Read the model definition and answer for the solid it produces. Units are mm, in the model's axes. Give positions to 0.01 mm unless a question says otherwise; leave off trailing zeros. Order: outer loops, then holes, each group sorted by start corner. A loop starts at its lowest first (then second) coordinate and runs counter-clockwise, first axis right, second up. Notation, with made-up numbers: M 66.5,13.25 L 90.5,13.25 A12 cw 90.5,24.25 Z; hole C 0,27 d6. An arc over 180 degrees is marked long. One line per item, written item: value.
from build123d import *

# Parameters (mm, degrees)
SKETCH1_W           = 210
SKETCH1_H           = 30
BOSS_EXTRUDE1_DEPTH = 3
SKETCH2_W           = 50
SKETCH2_H           = 3
BOSS_EXTRUDE2_DEPTH = 3
SKETCH3_R           = 8.15
CUT_EXTRUDE1_DEPTH  = 10
SKETCH4_R           = 2.5
CUT_EXTRUDE2_DEPTH  = 10


with BuildPart() as part:
    # Sketch1 → Boss-Extrude1 (new body)
    with BuildSketch(Plane(origin=(0, 0, 0), x_dir=(1, 0, 0), z_dir=(0, 1, 0))):
        Rectangle(SKETCH1_W, SKETCH1_H)
    extrude(amount=BOSS_EXTRUDE1_DEPTH)

    # Sketch2 → Boss-Extrude2 (add)
    with BuildSketch(Plane(origin=(0, 0, 0), x_dir=(1, 0, 0), z_dir=(0, 1, 0))):
        with Locations((-50, 16.5)):
            Rectangle(SKETCH2_W, SKETCH2_H)
        with Locations((50, 16.5)):
            Rectangle(SKETCH2_W, SKETCH2_H)
        with Locations((50, -16.5)):
            Rectangle(SKETCH2_W, SKETCH2_H)
        with Locations((-50, -16.5)):
            Rectangle(SKETCH2_W, SKETCH2_H)
    extrude(amount=BOSS_EXTRUDE2_DEPTH)

    # Sketch3 → Cut-Extrude1 (cut)
    with BuildSketch(Plane(origin=(0, 3, 0), x_dir=(1, 0, 0), z_dir=(0, 1, 0))):
        with Locations(Location((-12.7, 0, 0), (0, 0, 270))):
            Circle(SKETCH3_R)
        with Locations(Location((12.7, 0, 0), (0, 0, 90))):
            Circle(SKETCH3_R)
    extrude(amount=-CUT_EXTRUDE1_DEPTH, mode=Mode.SUBTRACT)

    # Sketch4 → Cut-Extrude2 (cut)
    with BuildSketch(Plane(origin=(0, 3, 0), x_dir=(1, 0, 0), z_dir=(0, 1, 0))):
        with Locations(Location((-95, 0, 0), (0, 0, 270))):
            Circle(SKETCH4_R)
        with Locations(Location((-87.5, 5, 0), (0, 0, 270))):
            Circle(SKETCH4_R)
        with Locations(Location((-87.5, -5, 0), (0, 0, 270))):
            Circle(SKETCH4_R)
        with Locations(Location((87.5, -5, 0), (0, 0, 90))):
            Circle(SKETCH4_R)
        with Locations(Location((87.5, 5, 0), (0, 0, 90))):
            Circle(SKETCH4_R)
        with Locations(Location((95, 0, 0), (0, 0, 90))):
            Circle(SKETCH4_R)
    extrude(amount=-CUT_EXTRUDE2_DEPTH, mode=Mode.SUBTRACT)


solid = part.part
1) Consider probe 1 along X at (y, z) = (1.9, 0); probe 2 along Z at (x, y) = (87.5, 1.3); probe 3 along X at (y, z) = (1.6, 16.5). Determine where each line is inside the solid, lowest interval first.
Reported:
probe 1: x = -105 to -97.5, -92.5 to -20.85, -4.55 to 4.55, 20.85 to 92.5, 97.5 to 105
probe 2: z = -15 to -7.5, -2.5 to 2.5, 7.5 to 15
probe 3: x = -75 to -25, 25 to 75
2) Find section B-B, the plane x = 87.5. Write down the section's boundary in (y, z).
Reported:
outline: M 0,-15 L 3,-15 L 3,-7.5 L 0,-7.5 Z; M 0,-2.5 L 3,-2.5 L 3,2.5 L 0,2.5 Z; M 0,7.5 L 3,7.5 L 3,15 L 0,15 Z
3) Find section A-A, the plane x = 12.7. Write down the section's boundary in (y, z), plus the area to 3 significant figures.
Reported:
outline: M 0,-15 L 3,-15 L 3,-8.15 L 0,-8.15 Z; M 0,8.15 L 3,8.15 L 3,15 L 0,15 Z
area: 41.1 mm^2
4) Find section D-D, the plane z = 5. Write down the section's boundary in (x, y).
Reported:
outline: M -105,0 L -90,0 L -90,3 L -105,3 Z; M -85,0 L -19.14,0 L -19.14,3 L -85,3 Z; M -6.26,0 L 6.26,0 L 6.26,3 L -6.26,3 Z; M 19.14,0 L 85,0 L 85,3 L 19.14,3 Z; M 90,0 L 105,0 L 105,3 L 90,3 Z
5) Find section C-C, the plane y = 2.15. Count the separate pieces of the cut face and the enclosed holes in it, plus the area to 3 significant figures.
Reported:
separate pieces: 1
enclosed holes: 8
area: 6,360 mm^2
6) Determine the mould class of faces 1 (the face through (-1, 3, 0)), 2 (the face through (-5.828, 1.521, 4.381)) for opening direction X: +X half, -X half, draft (parallel to the pull), parting line (faces both ways), or undercut.
Reported:
face 1: draft
face 2: undercut
7) Each of these flat-tipped pins is pushed along its axis until it touches: pin 1 Ø1.5 at (x, y) = (92.5, 2) entering from -Z; pin 2 Ø4 at (x, z) = (-87.5, -5) entering from +Y; pin 3 Ø1.5 at (y, z) = (2, 17) entering from -X; pin 4 Ø1.5 at (x, y) = (-83.5, 2) entering from +Z. Where does it stop, or does it pass through?
Reported:
pin 1: stops at z = -15
pin 2: passes through
pin 3: stops at x = -75
pin 4: stops at z = 15
